Input: part model. Units: mm. Frame: model coordinates. A direction names the side the tool comes from. Coordinates: 2 decimals unless noted, no trailing zeros. Loops run counter-clockwise (first coordinate to the right, second up) from the corner with the lowest first, then second, coordinate; pieces in that order, holes last. Notation, with made-up numbers: (-27.5, 25.25) -> (-22.5, 25.25) arc R19 cw to (-22.5, 51.25) -> close; hole circle Ø6 at (-21.75, 49). An arc over 180 degrees is marked (long way). Put each result on its own line as item: value. Start each with the question number.
1) Cut plane A-A (x = 87). Return the cut outline in (y, z), plus the area to 3 significant figures.
2) Cut plane B-B (z = 17). Return the cut outline in (x, y), plus the area to 3 significant figures.
3) Material intervals for L1, parallel to X at y = 20, z = 16; L2, parallel to Z at x = 17, y = 5; L3, parallel to Z at x = 46.5, y = 83.5, sorted ascending.
4) Set-up query: faces 4 (the flat face through (49.3, 22.739, 29.385)), 5 (the flat face through (49, -3, 5)), 6 (the flat face through (49.3, 53.11, 21.99)). Return all of +Z, -Z, +X, -X, +Y, -Y with unobstructed straight access to the full face (end or side cutting, diameter ignored); none if empty.
5) Pull-direction query (X, two-part tool) for faces 1 (the flat face through (5, 33, 22)), 2 (the flat face through (0, 37, 22)), 3 (the flat face through (49.3, 35.082, 55.694)); classes: pulls with the +X half, pulls with the -X half, needs draft (parallel to the pull), parting line crosses it, or undercut.
6) Cut plane C-C (y = 30). Return the cut outline in (x, z), plus the area to 3 significant figures.
7) Contact query for flat-ended pins moving along their axis: P1, Ø14, axis at x = 31, y = -5, coming from the +Z side; P2, Ø6, axis at x = 70, z = 45.5, coming from the +Y side (3 decimals); P3, Ø6, axis at x = 31.5, y = 44.5, coming from the +Z side; P4, Ø17, axis at y = 37, z = 14.5, coming from the -X side. Output: stop coordinate, or through.
8) Cut plane D-D (y = 14). Return the cut outline in (x, z), plus the area to 3 significant figures.
from build123d import *

# Parameters (mm, degrees)
F1_DEPTH = 100
F3_DEPTH = 5
F5_DEPTH = 5
F6_DEPTH = 10


with BuildPart() as f1:
    # F0 (on Right) → F1 (new body)
    with BuildSketch(Plane.YZ):
        Polygon((0, 5), (0, 0), (100, 0), (100, 5), (43.3012701892, 5), (63.1976404784, 39.4615242271), (57.4241377865, 39.4615242271), (37.5277674973, 5), (8.6602540378, 5), (37.2168783649, 54.4615242271), (32.8867513459, 56.9615242271), (2.8867513459, 5), align=None)
    extrude(amount=F1_DEPTH)

    # F2 (on face) → F3 (join)
    with BuildSketch(Plane.YZ.offset(100)):
        Polygon((37.5277674973, 5), (57.4241377865, 39.4615242271), (28.556624327, 39.4615242271), (8.6602540378, 5), align=None)
    extrude(amount=-F3_DEPTH)

    # F4 (on face) → F5 (join)
    with BuildSketch(Plane(origin=(0, 0, 0), x_dir=(0, -1, 0), z_dir=(-1, 0, 0))):
        Polygon((-28.556624327, 39.4615242271), (-57.4241377865, 39.4615242271), (-37.5277674973, 5), (-8.6602540378, 5), align=None)
    extrude(amount=-F5_DEPTH)

    # F6 (add): a face of the model
    f6_faces = [f1.faces().sort_by_distance(p)[0] for p in [
        (50, 0, 2.5),
    ]]
    extrude(f6_faces, amount=F6_DEPTH)


solid = f1.part
Results found:
1. outline: (-10, 0) -> (100, 0) -> (100, 5) -> (43.3, 5) -> (63.2, 39.46) -> (57.42, 39.46) -> (37.53, 5) -> (8.66, 5) -> (37.22, 54.46) -> (32.89, 56.96) -> (2.89, 5) -> (-10, 5) -> close
1. area: 1,040 mm2
2. outline: (0, 9.81) -> (100, 9.81) -> (100, 50.23) -> (0, 50.23) -> close; hole (5, 15.59) -> (95, 15.59) -> (95, 44.46) -> (5, 44.46) -> close
2. area: 1,440 mm2
3. L1: x = 0 to 5, 95 to 100
3. L2: z = 0 to 8.66
3. L3: z = 0 to 5
4. face 4: none
4. face 5: +Z, +X, -X, -Y
4. face 6: +X, -X, +Y
5. face 1: undercut
5. face 2: pulls with the -X half
5. face 3: needs draft
6. outline: (0, 0) -> (100, 0) -> (100, 39.46) -> (95, 39.46) -> (95, 5) -> (5, 5) -> (5, 39.46) -> (0, 39.46) -> close; (0, 41.96) -> (100, 41.96) -> (100, 51.96) -> (0, 51.96) -> close
6. area: 1,840 mm2
7. P1: stops at z = 5
7. P2: stops at y = 33.775
7. P3: stops at z = 22.27
7. P4: stops at x = 0
8. outline: (0, 0) -> (100, 0) -> (100, 24.25) -> (0, 24.25) -> close; hole (5, 5) -> (95, 5) -> (95, 14.25) -> (5, 14.25) -> close
8. area: 1,590 mm2
